```python
from build123d import *
from build123d.topology import SkipClean

# Parameters (mm, degrees)
SKETCH1_R           = 3.5
SKETCH1_R_2         = 2.5
BOSS_EXTRUDE1_DEPTH = 6.25
BOSS_EXTRUDE2_DEPTH = 1.3


with BuildPart() as part:
    # Sketch1 → Boss-Extrude1 (new body)
    with BuildSketch(Plane(origin=(0, 0, 0), x_dir=(1, 0, 0), z_dir=(0, 1, 0))):
        with Locations(Location((0, 0, 0), (0, 0, 270))):
            Circle(SKETCH1_R)
        with Locations(Location((0, 0, 0), (0, 0, 270))):
            Circle(SKETCH1_R_2, mode=Mode.SUBTRACT)
    extrude(amount=BOSS_EXTRUDE1_DEPTH)

    # Sketch2 → Boss-Extrude2 (add)
    with SkipClean():  # the faces are left unmerged after this step: merging them gives an invalid solid
        with BuildSketch(Plane(origin=(0, 6.25, 0), x_dir=(1, 0, 0), z_dir=(0, 1, 0))):
            with BuildLine():
                Line((2.344759123, 0.867239676), (3.282662772, 1.214135546))
                ThreePointArc((3.282662772, 1.214135546), (3.5, 0), (3.282662772, -1.214135546))
                Line((3.282662772, -1.214135546), (2.344759123, -0.867239676))
                ThreePointArc((2.344759123, -0.867239676), (2.5, 0), (2.344759123, 0.867239676))
            make_face()
            with BuildLine():
                Line((-2.344759123, -0.867239676), (-3.282662772, -1.214135546))
                ThreePointArc((-3.282662772, -1.214135546), (-3.5, 0), (-3.282662772, 1.214135546))
                Line((-3.282662772, 1.214135546), (-2.344759123, 0.867239676))
                ThreePointArc((-2.344759123, 0.867239676), (-2.5, 0), (-2.344759123, -0.867239676))
            make_face()
        extrude(amount=BOSS_EXTRUDE2_DEPTH)


solid = part.part
```
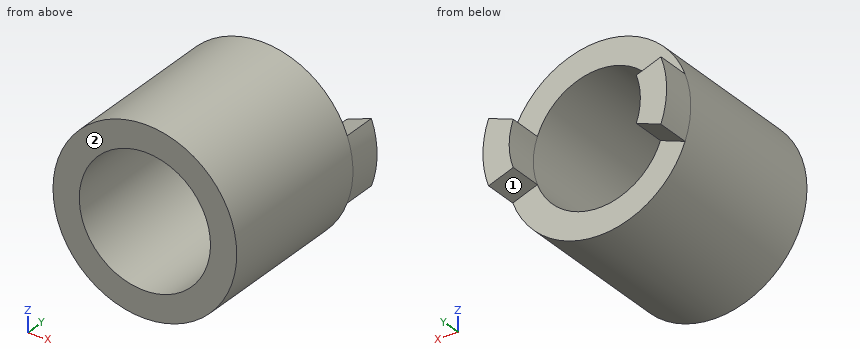
Input: part model. Units: mm. Frame: model coordinates. Face numbers are marked on the shaded views. Coordinates: 2 decimals unless noted, no trailing zeros. Write each loop counter-clockwise with the first axis right and the second up, starting at its lowest first coordinate (ties: lowest second). Pieces come first, ordered by that corner, then holes. Notation, with made-up numbers: (31, -18) -> (42, -18) arc R25 ccw to (42, -1) -> close; hole circle Ø1 at (-16, -36). An arc over 180 degrees is marked (long way). Answer as a JSON object with one key per item and string values.
1. Section C-C on y = 2.5. Return the cut outline in (x, z).
Result set:
{"outline": "circle Ø7 at (0, 0); hole circle Ø5 at (0, 0)"}
2. Mould query, pull axis X, two halves, no side actions, for the marked faces 1 and 2. Classes: released by +X, released by -X, zero draft, split by the parting line, or undercut.
Result set:
{"face 1": "undercut", "face 2": "zero draft"}
3. Section D-D on z = 1. Return the cut outline in (x, y), then the cut area to 3 significant figures.
Result set:
{"outline": "(-3.35, 0) -> (-2.29, 0) -> (-2.29, 6.25) -> (-2.7, 6.25) -> (-2.7, 7.55) -> (-3.35, 7.55) -> close; (2.29, 0) -> (3.35, 0) -> (3.35, 7.55) -> (2.7, 7.55) -> (2.7, 6.25) -> (2.29, 6.25) -> close", "area": "15.0 mm2"}
4. Section B-B on z = 0. Return the cut outline in (x, y).
Result set:
{"outline": "(-3.5, 0) -> (-2.5, 0) -> (-2.5, 7.55) -> (-3.5, 7.55) -> close; (2.5, 0) -> (3.5, 0) -> (3.5, 7.55) -> (2.5, 7.55) -> close"}
5. Section A-A on x = 0. Return the cut outline in (y, z).
Result set:
{"outline": "(0, -3.5) -> (6.25, -3.5) -> (6.25, -2.5) -> (0, -2.5) -> close; (0, 2.5) -> (6.25, 2.5) -> (6.25, 3.5) -> (0, 3.5) -> close"}
6. First-contact query: P1, Ø0.8, axis at x = -1, z = -2.5, coming from the +Y side. Flat tip, straight axial feed; report the tip coordinate or a pass-through.
Result set:
{"P1": "stops at y = 6.25"}
7. Material intervals for line 1 (X direction, y = 4, z = 0); line 2 (Y direction, x = -2.75, z = -1.5); line 3 (X direction, y = 5, z = 1.25), sorted ascending. Write a range as from..to.
Result set:
{"line 1": "x = -3.5..-2.5, 2.5..3.5", "line 2": "y = 0..6.25", "line 3": "x = -3.27..-2.17, 2.17..3.27"}
